Geometry: final body of the model. Coordinates: model frame, mm. A direction names the side the tool comes from. Give positions to 0.01 mm unless a question says otherwise; leave off trailing zeros. Answer in a Markdown table with one row per item. Add a question column.
Item 1: Access query for faces 5 (the cylindrical face through (6.89, 72.1, -85.57)), 6 (the cylindrical face through (-106.263, 34.989, -100.182)), 7 (the cylindrical face through (-91.8, 35.34, -100.18)). Directions: +Z, -Z, +X, -X, +Y, -Y. A direction counts if a zero-diameter tool reaches every point of the face in a straight line with its end or side. Return the directions, or none.
Item 2: Draft query along Y for faces 1 (the flat face through (111.682, 59.577, -99.818)), 2 (the flat face through (-93.95, 14.09, -100.18)), 3 (the flat face through (25, 81, -115)), 4 (the cylindrical face through (8.5, 81.9, -85.6)). Return one class per face: +Y half, -Y half, draft (parallel to the pull), parting line (faces both ways), or undercut.
Item 3: First-contact query: P1, Ø8, axis at y = 47.5, z = -98.5, coming from the -X side; P2, Ø4, axis at x = 35.5, z = -89.5, coming from the +Y side; P3, Ø1.5, axis at x = 10.5, y = 1.5, coming from the +Z side. Flat tips, straight axial feed; report the tip coordinate or a pass-through.
Item 4: Material intervals for probe 1 along Y at (x, z) = (-84, -106.5); probe 2 along Y at (x, z) = (95, -108); probe 3 along X at (y, z) = (19, -107.5), sorted ascending. Write a range as from..to.
```python
from build123d import *

# Parameters (mm, degrees)
SKETCH2_W           = 250
SKETCH2_H           = 30
BOSS_EXTRUDE1_DEPTH = 10
SKETCH3_W           = 5
SKETCH3_H           = 30
BOSS_EXTRUDE2_DEPTH = 10
SKETCH4_W           = 200
SKETCH4_H           = 30
BOSS_EXTRUDE3_DEPTH = 6
SKETCH11_W          = 30
SKETCH11_H          = 55
CUT_EXTRUDE2_DEPTH  = 10
FILLET1_R           = 25
FILLET9_R           = 10
FILLET8_R           = 10
FILLET11_R          = 25
FILLET5_R           = 6
FILLET10_R          = 100
FILLET6_R           = 2
SKETCH12_W          = 20
SKETCH12_H          = 20
SKETCH12_W_2        = 5
SKETCH12_H_2        = 7.5
CUT_EXTRUDE3_DEPTH  = 3


with BuildPart() as part:
    # Sketch2 → Boss-Extrude1 (new body)
    with BuildSketch(Plane(origin=(-23.43534086, 72.126562752, 0), x_dir=(0.9510565162951534, 0.3090169943749482, 0), z_dir=(-0.3090169943749481, 0.9510565162951533, 0))):
        with Locations((33.98053096, 100)):
            Rectangle(SKETCH2_W, SKETCH2_H)
    extrude(amount=-BOSS_EXTRUDE1_DEPTH)

    # Sketch3 → Boss-Extrude2 (add)
    with BuildSketch(Plane(origin=(-23.43534086, 72.126562752, 0), x_dir=(0.9510565162951534, 0.3090169943749482, 0), z_dir=(-0.3090169943749481, 0.9510565162951533, 0))):
        with Locations((-88.51946904, 100)):
            Rectangle(SKETCH3_W, SKETCH3_H)
    extrude(amount=BOSS_EXTRUDE2_DEPTH)



with BuildPart() as body_2:
    # Sketch4 → Boss-Extrude3 (new body)
    with BuildSketch(Plane(origin=(0, 0, 0), x_dir=(1, 0, 0), z_dir=(0, 1, 0))):
        with Locations((15, 100)):
            Rectangle(SKETCH4_W, SKETCH4_H)
    extrude(amount=BOSS_EXTRUDE3_DEPTH)


with BuildPart() as part_1:
    add(part.part)

    add(body_2.part)  # Loft1 merges body 2
    # Sketch6 → Loft1 section 0
    with BuildSketch(Plane(origin=(-23.43534086, 72.126562752, 0), x_dir=(0.9510565162951534, 0.3090169943749482, 0), z_dir=(0.3090169943749481, -0.9510565162951533, 0))):
        with BuildLine():
            Line((158.98053096, -85), (148.98053096, -85))
            Line((148.98053096, -85), (148.98053096, -115))
            Line((148.98053096, -115), (158.98053096, -115))
            Line((158.98053096, -115), (158.98053096, -85))
        make_face()
    # Sketch5 → Loft1 section 1
    with BuildSketch(Plane(origin=(0, 0, 0), x_dir=(1, 0, 0), z_dir=(0, 1, 0))):
        with BuildLine():
            Line((115, 115), (105, 115))
            Line((105, 115), (105, 85))
            Line((105, 85), (115, 85))
            Line((115, 85), (115, 115))
        make_face()
    loft()

    # Sketch11 → Cut-Extrude2 (cut)
    with BuildSketch(Plane(origin=(113.739623688, -11.973083454, 0), x_dir=(0, 0, -1), z_dir=(0.9945050055104876, -0.1046890348345292, 0))):
        with Locations((100, 135.5)):
            Rectangle(SKETCH11_W, SKETCH11_H)
    extrude(amount=CUT_EXTRUDE2_DEPTH, mode=Mode.SUBTRACT)

    # Sketch9 → Loft2 section 0
    with BuildSketch(Plane(origin=(-20.345170916, 62.615997589, 0), x_dir=(0.9510565162951534, 0.3090169943749482, 0), z_dir=(0.3090169943749481, -0.9510565162951533, 0))):
        with BuildLine():
            Line((-91.01946904, -85), (-81.01946904, -85))
            Line((-81.01946904, -85), (-81.01946904, -115))
            Line((-81.01946904, -115), (-91.01946904, -115))
            Line((-91.01946904, -115), (-91.01946904, -85))
        make_face()
    # Sketch10 → Loft2 section 1
    with BuildSketch(Plane(origin=(0, 0, 0), x_dir=(1, 0, 0), z_dir=(0, 1, 0))):
        with BuildLine():
            Line((-85, 115), (-75, 115))
            Line((-75, 115), (-75, 85))
            Line((-75, 85), (-85, 85))
            Line((-85, 85), (-85, 115))
        make_face()
    loft()

    # Fillet1
    fillet1_edges = [part_1.edges().sort_by_distance(p)[0] for p in [
        (105.672974261, 6, -100),
        (-78.576290654, 6, -100),
    ]]
    fillet(fillet1_edges, radius=FILLET1_R)

    # Fillet9
    fillet9_edges = [part_1.edges().sort_by_distance(p)[0] for p in [
        (127.764129074, 121.254248594, -100),
    ]]
    fillet(fillet9_edges, radius=FILLET9_R)

    # Fillet8
    fillet8_edges = [part_1.edges().sort_by_distance(p)[0] for p in [
        (117.029613529, 107.251770821, -100),
        (-97.399264893, 37.579604781, -100),
        (-85, 0, -100),
    ]]
    fillet(fillet8_edges, radius=FILLET8_R)

    # Fillet11
    fillet11_edges = [part_1.edges().sort_by_distance(p)[0] for p in [
        (115, 0, -100),
    ]]
    fillet(fillet11_edges, radius=FILLET11_R)

    # Fillet5
    fillet5_edges = [part_1.edges().sort_by_distance(p)[0] for p in [
        (-105.244717419, 45.545084972, -100),
    ]]
    fillet(fillet5_edges, radius=FILLET5_R)

    # Fillet10
    fillet10_edges = [part_1.edges().sort_by_distance(p)[0] for p in [
        (-106.909830056, 34.489434837, -100),
    ]]
    fillet(fillet10_edges, radius=FILLET10_R)

    # Fillet6
    fillet6_edges = [part_1.edges().sort_by_distance(p)[0] for p in [
        (9.473412371, 6, -115),
        (9.473412371, 6, -85),
        (-76.722563068, 9.262951119, -85),
        (-76.722563068, 9.262951119, -115),
        (99.983633439, 12.363146047, -85),
        (99.983633439, 12.363146047, -115),
        (121.753976282, 64.160140842, -85),
        (121.753976282, 64.160140842, -115),
        (6.789088019, 81.947075002, -85),
        (122.500555572, 114.755349451, -85),
        (122.500555572, 114.755349451, -115),
        (6.494058609, 0, -85),
        (-88.417020392, 22.509949594, -85),
        (8.392983609, 71.953590028, -85),
        (111.732266775, 60.02250459, -85),
        (-84.320965292, 1.235829976, -85),
        (8.392983609, 71.953590028, -115),
        (-88.417020392, 22.509949594, -115),
        (111.732266775, 60.02250459, -115),
        (-84.320965292, 1.235829976, -115),
        (-91.756560464, 35.458482469, -85),
        (-91.756560464, 35.458482469, -115),
        (111.682636246, 100.69569196, -115),
        (111.682636246, 100.69569196, -85),
        (-107.716853374, 53.153537102, -85),
        (-107.716853374, 53.153537102, -115),
        (-113.090169944, 53.510565163, -100),
        (-110.712528653, 54.283107649, -85),
        (-108.334887362, 55.055650135, -100),
        (6.494058609, 0, -115),
        (109.220318345, 6.420028972, -115),
        (-110.712528653, 54.283107649, -115),
        (109.220318345, 6.420028972, -85),
        (6.789088019, 81.947075002, -115),
        (-104.116423285, 47.759486891, -115),
        (-104.116423285, 47.759486891, -85),
        (-111.955491831, 50.018385015, -85),
        (-111.955491831, 50.018385015, -115),
        (-94.034829619, 14.222208325, -85),
        (-106.188112518, 34.829251267, -85),
        (-94.034829619, 14.222208325, -115),
        (-106.188112518, 34.829251267, -115),
    ]]
    fillet(fillet6_edges, radius=FILLET6_R)

    # Sketch12 → Cut-Extrude3 (cut)
    with BuildSketch(Plane.XZ):
        with Locations((7.494564149, -95)):
            Rectangle(SKETCH12_W, SKETCH12_H)
        with Locations((7.494564149, -95)):
            Rectangle(SKETCH12_W_2, SKETCH12_H_2, mode=Mode.SUBTRACT)
    extrude(amount=-CUT_EXTRUDE3_DEPTH, mode=Mode.SUBTRACT)


solid = part_1.part
```
Findings below:
| question | item | result |
|---|---|---|
| 1 | face 5 | +Z |
| 1 | face 6 | +Z, -Z, -X, -Y |
| 1 | face 7 | +Z, -Z |
| 2 | face 1 | undercut |
| 2 | face 2 | -Y half |
| 2 | face 3 | draft |
| 2 | face 4 | +Y half |
| 3 | P1 | stops at x = -112.44 |
| 3 | P2 | stops at y = 91.93 |
| 3 | P3 | stops at z = -91.25 |
| 4 | probe 1 | y = 1.07..15.51, 41.93..52.45 |
| 4 | probe 2 | y = 0.13..8.9, 100.09..110.61 |
| 4 | probe 3 | x = -97.07..-86.32, 105.25..116.76 |
